Geometry check sheet. Reference: drawing and pictorial views, mm from the part's lowest x, y, z. A direction names the side the tool comes from. Give positions to 0.01 mm unless a question says otherwise; leave off trailing zeros. Loops run counter-clockwise (first coordinate to the right, second up) from the corner with the lowest first, then second, coordinate; pieces in that order, holes last. Notation, with made-up numbers: (-5.5, 5.5) -> (36.5, 5.5) arc R20 cw to (36.5, 11.5) -> close; hole circle Ø2 at (-14, 67.25). An arc over 180 degrees is marked (long way). Answer in a Markdown table with one row per item. Add a question column.
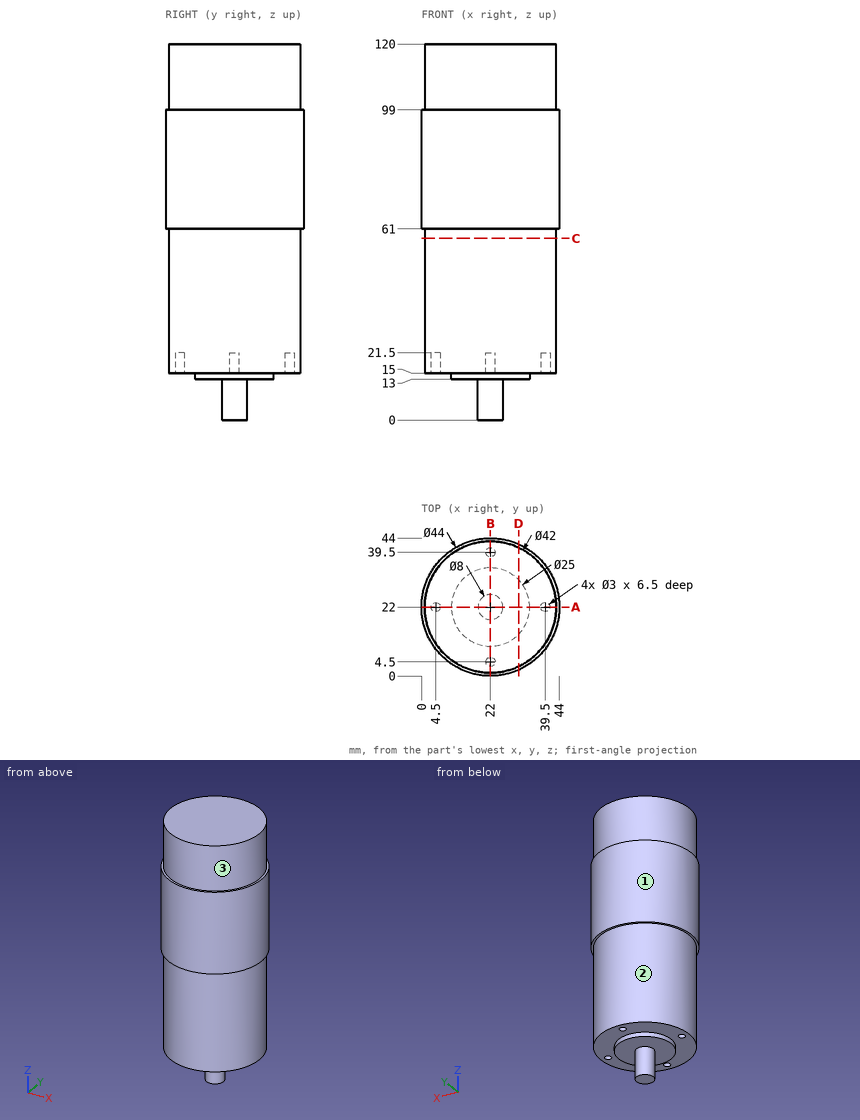
1. Gauge pin test, flat ends, axial feed: pin 1 Ø1.5 at (x, y) = (4, 21.5) entering from -Z; pin 2 Ø4 at (x, y) = (6, 13) entering from -Z; pin 3 Ø1 at (y, z) = (11, 25) entering from +X; pin 4 Ø12.5 at (x, y) = (27, 24.5) entering from -Z. Record the tip position at first contact, or that the pin passes through.
2. Sectioned sample at A-A (y = 22). Enter the section's corners in (x, z), plus the area to 3 significant figures.
3. Sectioned sample at D-D (x = 31). Enter the section's corners in (y, z), plus the area to 3 significant figures.
4. Access from +Z, -Z, +X, -X, +Y, -Y to the whole of each face (thin tool, end or side, straight path). Record for the marked faces 1, 2 and 3.
5. Material ranges on L1, parallel to X at y = 22, z = 20.25; L2, parallel to Y at x = 21, z = 20.5, recorded low to high. Write a range as from..to.
6. Sectioned sample at C-C (z = 58). Enter the section's corners in (x, y), plus the area to 3 significant figures.
Response:
| question | item | result |
|---|---|---|
| 1 | pin 1 | stops at z = 21.5 |
| 1 | pin 2 | stops at z = 15 |
| 1 | pin 3 | stops at x = 40.19 |
| 1 | pin 4 | stops at z = 0 |
| 2 | outline | (0, 61) -> (1, 61) -> (1, 15) -> (3, 15) -> (3, 21.5) -> (6, 21.5) -> (6, 15) -> (9.5, 15) -> (9.5, 13) -> (18, 13) -> (18, 0) -> (26, 0) -> (26, 13) -> (34.5, 13) -> (34.5, 15) -> (38, 15) -> (38, 21.5) -> (41, 21.5) -> (41, 15) -> (43, 15) -> (43, 61) -> (44, 61) -> (44, 99) -> (43, 99) -> (43, 120) -> (1, 120) -> (1, 99) -> (0, 99) -> close |
| 2 | area | 4,600 mm2 |
| 3 | outline | (1.93, 61) -> (3.03, 61) -> (3.03, 15) -> (13.33, 15) -> (13.33, 13) -> (30.67, 13) -> (30.67, 15) -> (40.97, 15) -> (40.97, 61) -> (42.07, 61) -> (42.07, 99) -> (40.97, 99) -> (40.97, 120) -> (3.03, 120) -> (3.03, 99) -> (1.93, 99) -> close |
| 3 | area | 4,100 mm2 |
| 4 | face 1 | +Z, -Z |
| 4 | face 2 | -Z |
| 4 | face 3 | +Z |
| 5 | L1 | x = 1..3, 6..38, 41..43 |
| 5 | L2 | y = 1.02..3.38, 5.62..38.38, 40.62..42.98 |
| 6 | outline | circle Ø42 at (22, 22) |
| 6 | area | 1,390 mm2 |
